The drawing under review shows one solid part. Ordinate dimensions are in mm from its lowest x, y, z. A direction names the side the tool comes from. Give positions to 0.01 mm unless a question says otherwise; leave off trailing zeros. Loops run counter-clockwise (first coordinate to the right, second up) from the corner with the lowest first, then second, coordinate; pieces in that order, holes last. Notation, with made-up numbers: (25, 18) - (77, 18) arc R17 cw to (77, 26) - close; hole circle Ø9 at (89, -0.75). An arc over 180 degrees is marked (long way). Answer as CSV lines item,"result".
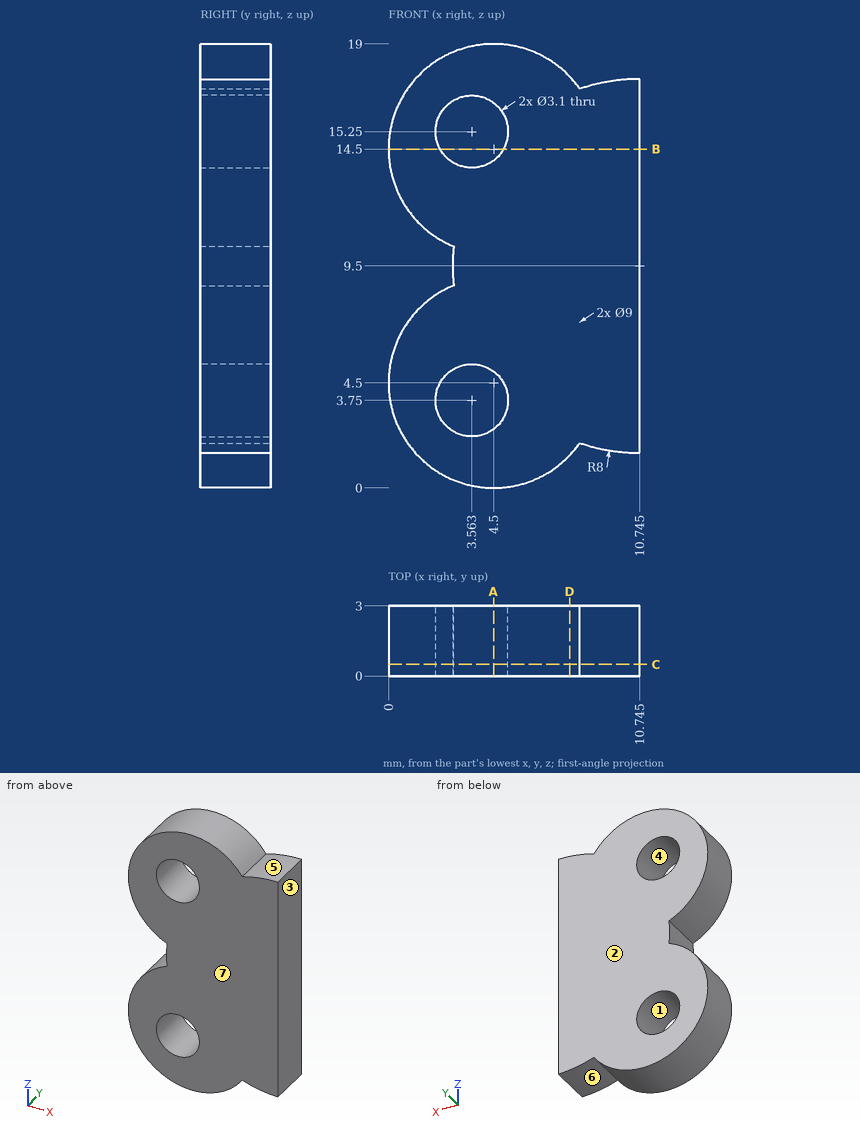
1) Consider section B-B on z = 14.5. Write out the cut boundary in (x, y) (1 decimal), and give its area (3 significant figures).
From the geometry:
outline,"(0, 0) - (2.2, 0) - (2.2, 3) - (0, 3) - close; (4.9, 0) - (10.7, 0) - (10.7, 3) - (4.9, 3) - close"
area,"24.1 mm^2"
2) Consider section A-A on x = 4.5. Write out the cut boundary in (y, z) (1 decimal).
From the geometry:
outline,"(0, 0) - (3, 0) - (3, 2.5) - (0, 2.5) - close; (0, 5) - (3, 5) - (3, 14) - (0, 14) - close; (0, 16.5) - (3, 16.5) - (3, 19) - (0, 19) - close"
3) Draft analysis for pull direction X (two halves, no side actions). For the marked faces 1, 2, 3 and 4, state which applies: pulls with the +X half, pulls with the -X half, needs draft (parallel to the pull), parting line crosses it, or undercut.
From the geometry:
face 1,"undercut"
face 2,"needs draft"
face 3,"pulls with the +X half"
face 4,"undercut"
4) Consider section C-C on y = 0.5. Count the separate pieces of the cut face and the enclosed holes in it, and give its area (3 significant figures).
From the geometry:
separate pieces,"1"
enclosed holes,"2"
area,"157 mm^2"
5) Consider section D-D on x = 7.75. Write out the cut boundary in (y, z).
From the geometry:
outline,"(0, 1.39) - (3, 1.39) - (3, 17.61) - (0, 17.61) - close"
6) Machinability: for the marked faces 5, 6 and 7, which of the approach directions +Z, -Z, +X, -X, +Y, -Y give a long, thin tool a straight path to every point of the face, cutting with its end or side? Answer none if there is none.
From the geometry:
face 5,"+Z, +Y, -Y"
face 6,"-Z, +Y, -Y"
face 7,"+Z, -Z, +X, -X, -Y"
7) Insertion check: P1, Ø5, axis at x = 5.5, z = 11, coming from the -Y side. The pin has a flat end and moves straight along its axis. Give the tip position at first contact, or say it passes through.
From the geometry:
P1,"stops at y = 0"
8) Wall thickness on line 1 (Z direction, x = 3.5, y = 2.45); line 2 (Z direction, x = 4.75, y = 0.8); line 3 (Z direction, x = 0.5, y = 2.1): over which ranges is each line inside the solid? List them lowest first. Write a range as from..to.
From the geometry:
line 1,"z = 0.11..2.2, 5.3..13.7, 16.8..18.89"
line 2,"z = 0.01..2.75, 4.75..14.25, 16.25..18.99"
line 3,"z = 2.44..6.56, 12.44..16.56"
